Autodesk Inventor part; units mm, degrees
ref_plane "YZ Plane" through (0, 0, 0) normal (1, 0, 0) x (0, 1, 0)
ref_plane "XZ Plane" through (0, 0, 0) normal (0, 1, 0) x (-1, 0, 0)
ref_plane "XY Plane" through (0, 0, 0) normal (0, 0, 1) x (1, 0, 0)
sketch "Sketch1" plane through (0, 0, 0) normal (0, 0, 1) x (1, 0, 0)
  line L0 (-47.0946, 30.5405) -> (-47.0946, -23.1081)
  line L1 (-47.0946, -23.1081) -> (50.0676, -23.1081)
  line L2 (50.0676, -23.1081) -> (50.0676, -13.1081)
  line L3 (50.0676, -13.1081) -> (-37.0946, -13.1081)
  line L4 (-37.0946, -13.1081) -> (-37.0946, 30.5405)
  line L5 (-37.0946, 30.5405) -> (-47.0946, 30.5405)
  point P0 (0, 0)
  dimension "d0" = 10
  dimension "d1" = 10
extrude "Extrusion1" add sketch "Sketch1" against normal blind 60
sketch "Sketch2" plane through (-47.0946, -23.1081, 0) normal (-1, 0, 0) x (0, 0, 1)
  line L0 (-60, 0) -> (-60, 53.6486)
  line L1 (0, 53.6486) -> (-60, 53.6486)
  line L2 (-45, 53.6486) -> (-45, 23.6486)
  line L3 (-45, 23.6486) -> (-15, 23.6486)
  line L4 (-15, 23.6486) -> (-15, 53.6486)
  point P0 (0, 23.1081)
  dimension "d4" = 15
  dimension "d5" = 15
  dimension "d6" = 30
  dimension "d7" = 30
extrude "Extrusion2" cut sketch "Sketch2" against normal blind 40
fillet "Fillet1" radius 15 2 edges at (-42.0946, 0.5405, -45) (-42.0946, 0.5405, -15)
sketch "Sketch3" plane through (-37.0946, -13.1081, 0) normal (0, 1, 0) x (1, 0, 0)
  line L0 (-10, 0) -> (87.1622, 0)
  line L1 (47.1622, 0) -> (47.1622, 15)
  line L2 (47.1622, 15) -> (67.1622, 15)
  line L3 (67.1622, 15) -> (67.1622, 0)
  point P0 (37.0946, 0)
  dimension "d11" = 20
  dimension "d12" = 20
  dimension "d13" = 15
extrude "Extrusion3" cut sketch "Sketch3" against normal through all
For this review, take the finished solid that the model builds, in its own axes (mm). A direction names the side the tool comes from. Round coordinates to 2 decimals unless told otherwise and drop trailing zeros. Write each loop counter-clockwise with the first axis right and the second up, starting at its lowest first coordinate (ties: lowest second). Pieces come first, ordered by that corner, then holes. Notation, with made-up numbers: (52, 38.25) - (58, 38.25) arc R13 cw to (58, 44.25) - close; hole circle Ø10 at (82, 37). An arc over 180 degrees is marked (long way). Answer as CSV lines item,"result". Start each with the question number.
(1) Add section C-C, the plane y = -18. State the section outline as (x, z) points, plus the area to 3 significant figures.
(2) Add section D-D, the plane z = -50.5. State the section outline as (x, y) points.
(3) For line 1 (Y direction, x = 21, z = -23); line 2 (X direction, y = 9, z = -7); line 3 (Y direction, x = -39.5, z = -35), list the stretches that pass through material, from the lowest coordinate up.
(4) Add section B-B, the plane y = 20. State the section outline as (x, z) points, plus the area to 3 significant figures.
(5) For pin 1 (2 mm diameter, centred on x = 21, z = -34, fed in from +Y); pin 2 (1.5 mm diameter, centred on y = 19.5, z = -47.5, fed in from +X); pin 3 (8 mm diameter, centred on x = 21, y = -18, fed in from +Z), all flat-tipped, find the tip position at first contact; note any pin that passes through.
(6) Mouldability with a two-part tool opening along X and no side actions: class faces 1 (the flat face through (10.068, -18, -7)), 2 (the flat face through (-47.095, -2, -30)), 3 (the flat face through (20, -18, -15)), 4 (the flat face through (7, -13.108, -30)) as +X half, -X half, draft (parallel to the pull), parting line (faces both ways), or undercut.
(7) Machinability: for faces 5 (the cylindrical face through (-42.02, 5.05, -19.28)), 6 (the flat face through (40, -18, 0)), 7 (the flat face through (30.068, -18, -8)), 8 (the flat face through (50.068, -18, -30)), 9 (the flat face through (-37.095, -1, -30)), which of the approach directions +Z, -Z, +X, -X, +Y, -Y give a long, thin tool a straight path to every point of the face, cutting with its end or side? Answer none if there is none.
(8) Add section A-A, the plane z = -11. State the section outline as (x, y) points.
From the geometry:
1,outline,"(-47.09, -60) - (50.07, -60) - (50.07, 0) - (30.07, 0) - (30.07, -15) - (10.07, -15) - (10.07, 0) - (-47.09, 0) - close"
1,area,"5,530 mm²"
2,outline,"(-47.09, -23.11) - (50.07, -23.11) - (50.07, -13.11) - (-37.09, -13.11) - (-37.09, 30.54) - (-47.09, 30.54) - close"
3,line 1,"y = -23.11 to -13.11"
3,line 2,"x = -47.09 to -37.09"
3,line 3,"y = -23.11 to 1.4"
4,outline,"(-47.09, -60) - (-37.09, -60) - (-37.09, -45) - (-47.09, -45) - close; (-47.09, -15) - (-37.09, -15) - (-37.09, 0) - (-47.09, 0) - close"
4,area,"300 mm²"
5,pin 1,"stops at y = -13.11"
5,pin 2,"stops at x = -37.09"
5,pin 3,"stops at z = -15"
6,face 1,"undercut"
6,face 2,"-X half"
6,face 3,"undercut"
6,face 4,"draft"
7,face 5,"+X, -X, +Y"
7,face 6,"+Z, +X, -X, +Y, -Y"
7,face 7,"+Z, +Y, -Y"
7,face 8,"+Z, -Z, +X, +Y, -Y"
7,face 9,"+Z, -Z, +X, +Y"
8,outline,"(-47.09, -23.11) - (10.07, -23.11) - (10.07, -13.11) - (-37.09, -13.11) - (-37.09, 30.54) - (-47.09, 30.54) - close; (30.07, -23.11) - (50.07, -23.11) - (50.07, -13.11) - (30.07, -13.11) - close"
